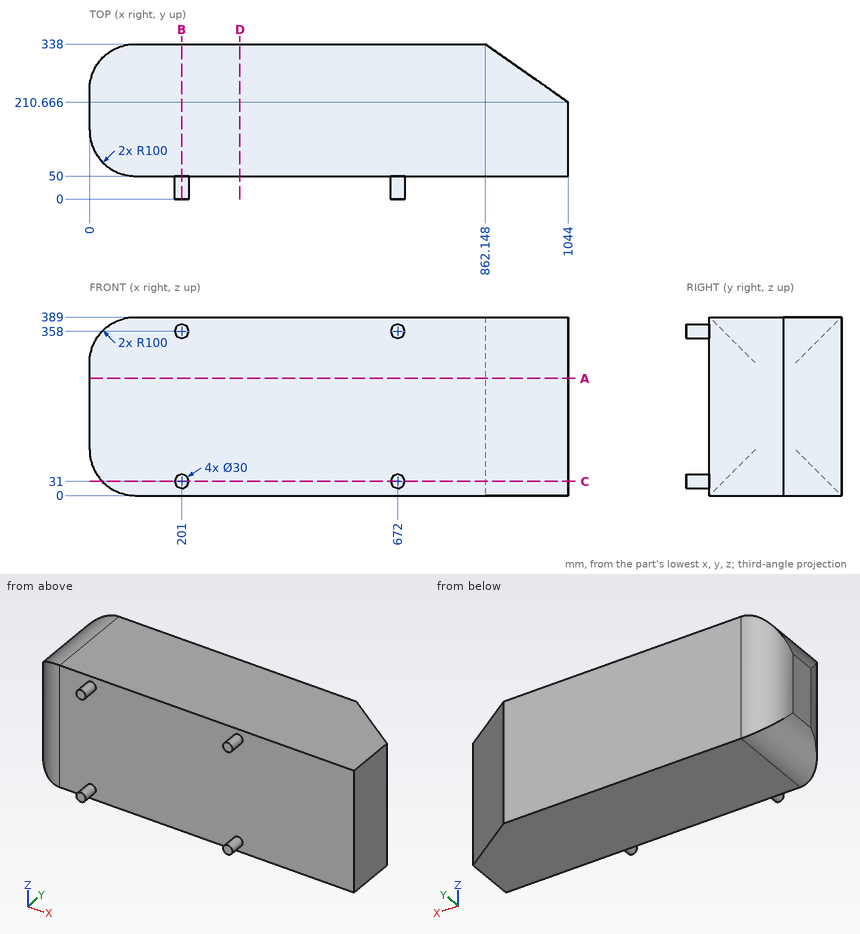
Design review of the part shown in the three views and the two pictorial views. Dimensions are in mm from the part's minimum x, y and z. Give positions to 0.01 mm unless a question says otherwise; leave off trailing zeros. Loops run counter-clockwise (first coordinate to the right, second up) from the corner with the lowest first, then second, coordinate; pieces in that order, holes last. Notation, with made-up numbers: M 8,69 L 34,69 A11 ccw 34,79 Z; hole C 37,-12 d10. An arc over 180 degrees is marked long. Write item = value, one per line.
Q1. We need section D-D (x = 328). Give the boundary of the cut face in (y, z), plus the area to 3 significant figures.
Output values:
outline = M 50,0 L 338,0 L 338,389 L 50,389 Z
area = 112,000 mm^2
Q2. We need section A-A (z = 255.5). Give the boundary of the cut face in (x, y).
Output values:
outline = M 0,150 A100 ccw 100,50 L 1044,50 L 1044,210.67 L 862.15,338 L 100,338 A100 ccw 0,238 Z
Q3. Insertion check: pin 1 (3 mm diameter, centred on x = 258.5, z = 271.5, fed in from -Y); pin 2 (12 mm diameter, centred on y = 43.5, z = 346, fed in from -X); pin 3 (6 mm diameter, centred on y = 69.5, z = 285, fed in from -X) (1 decimal). Each pin has a flat end and moves straight along its axis. Give the tip position at first contact, or say it passes through.
Output values:
pin_1 = 50
pin_2 = 187.25
pin_3 = 36.8
Q4. We need section C-C (z = 31). Give the boundary of the cut face in (x, y).
Output values:
outline = M 27.62,81 A100 ccw 100,50 L 186,50 L 186,0 L 216,0 L 216,50 L 657,50 L 657,0 L 687,0 L 687,50 L 1044,50 L 1044,210.67 L 862.15,338 L 100,338 A100 ccw 27.62,307 Z
Q5. To check wall thickness, follow line 1 (Y direction, x = 261, z = 65); line 2 (X direction, y = 95.5, z = 281); line 3 (X direction, y = 305, z = 161) (1 decimal). State the ranges of each line that lie inside material, in increasing order. Write a range as [from, to].
Output values:
line_1 = [50, 338]
line_2 = [16.16, 1044]
line_3 = [25.8, 909.3]
Q6. We need section B-B (x = 201). Give the boundary of the cut face in (y, z), plus the area to 3 significant figures.
Output values:
outline = M 0,16 L 50,16 L 50,0 L 338,0 L 338,389 L 50,389 L 50,373 L 0,373 L 0,343 L 50,343 L 50,46 L 0,46 Z
area = 115,000 mm^2
